```python
from build123d import *

# Parameters (mm, degrees)
BOSS_EXTRUDE3_DEPTH  = 125
SKETCH3_W            = 125
SKETCH3_H            = 92.089876837
BOSS_EXTRUDE5_DEPTH  = 12
CUT_EXTRUDE1_DEPTH   = 126
SKETCH7_W            = 105
SKETCH7_H            = 10
BOSS_EXTRUDE6_DEPTH  = 8
SKETCH8_W            = 105
SKETCH8_H            = 10
BOSS_EXTRUDE7_DEPTH  = 8
SKETCH9_W            = 105
SKETCH9_H            = 73.296024421
CUT_EXTRUDE2_DEPTH   = 16.420201433
SKETCH11_W           = 10
SKETCH11_H           = 73.296024421
CUT_EXTRUDE3_DEPTH   = 6
SKETCH12_W           = 10
SKETCH12_H           = 73.296024421
CUT_EXTRUDE4_DEPTH   = 6
SKETCH13_W           = 105
SKETCH13_H           = 32.67757118
CUT_EXTRUDE6_DEPTH   = 3
SKETCH14_R           = 1.9
CUT_EXTRUDE8_DEPTH   = 6
SKETCH15_R           = 1.9
CUT_EXTRUDE9_DEPTH   = 6
BOSS_EXTRUDE9_REACH  = 117
SKETCH25_W           = 10
SKETCH25_H           = 6
BOSS_EXTRUDE13_DEPTH = 10
CUT_EXTRUDE10_DEPTH  = 1
CUT_EXTRUDE11_DEPTH  = 1


with BuildPart() as part:
    # Sketch1 → Boss-Extrude3 (new body)
    with BuildSketch(Plane(origin=(0, 0, 0), x_dir=(0, 0, -1), z_dir=(1, 0, 0))):
        Polygon((0, 0), (92.089876837, 0), (0, 33.517974046), align=None)
    extrude(amount=-BOSS_EXTRUDE3_DEPTH)

    # Sketch3 → Boss-Extrude5 (add)
    with BuildSketch(Plane.XZ):
        with Locations((-62.5, -46.044938419)):
            Rectangle(SKETCH3_W, SKETCH3_H)
    extrude(amount=BOSS_EXTRUDE5_DEPTH)

    # Sketch6 → Cut-Extrude1 (cut, through all)
    with BuildSketch(Plane.ZY.offset(125)):
        Polygon((-9.396926208, 30.097772613), (-82.692950629, 3.420201433), (-9.396926208, 3.420201433), align=None)
    extrude(amount=-CUT_EXTRUDE1_DEPTH, mode=Mode.SUBTRACT)

    # Sketch7 → Boss-Extrude6 (add)
    with BuildSketch(Plane(origin=(0, 29.597115904, -10.772469209), x_dir=(1, 0, 0), z_dir=(0, 0.939692621, -0.342020143))):
        with Locations((-62.5, 81.536177713)):
            Rectangle(SKETCH7_W, SKETCH7_H)
    extrude(amount=BOSS_EXTRUDE6_DEPTH)

    # Sketch8 → Boss-Extrude7 (add)
    with BuildSketch(Plane(origin=(0, 29.597115904, -10.772469209), x_dir=(1, 0, 0), z_dir=(0, 0.939692621, -0.342020143))):
        with Locations((-62.5, -6.463822287)):
            Rectangle(SKETCH8_W, SKETCH8_H)
    extrude(amount=BOSS_EXTRUDE7_DEPTH)

    # Sketch9 → Cut-Extrude2 (cut, through all)
    with BuildSketch(Plane(origin=(0, 3.420201433, 0), x_dir=(1, 0, 0), z_dir=(0, 1, 0))):
        with Locations((-62.5, 46.044938419)):
            Rectangle(SKETCH9_W, SKETCH9_H)
    extrude(amount=-CUT_EXTRUDE2_DEPTH, mode=Mode.SUBTRACT)

    # Sketch11 → Cut-Extrude3 (cut)
    with BuildSketch(Plane(origin=(0, 3.420201433, 0), x_dir=(1, 0, 0), z_dir=(0, 1, 0))):
        with Locations((-5, 46.044938419)):
            Rectangle(SKETCH11_W, SKETCH11_H)
    extrude(amount=-CUT_EXTRUDE3_DEPTH, mode=Mode.SUBTRACT)

    # Sketch12 → Cut-Extrude4 (cut)
    with BuildSketch(Plane(origin=(0, 3.420201433, 0), x_dir=(1, 0, 0), z_dir=(0, 1, 0))):
        with Locations((-120, 46.044938419)):
            Rectangle(SKETCH12_W, SKETCH12_H)
    extrude(amount=-CUT_EXTRUDE4_DEPTH, mode=Mode.SUBTRACT)

    # Sketch13 → Cut-Extrude6 (cut)
    with BuildSketch(Plane(origin=(0, 0, -9.396926208), x_dir=(-1, 0, 0), z_dir=(0, 0, -1))):
        with Locations((62.5, 13.758987023)):
            Rectangle(SKETCH13_W, SKETCH13_H)
    extrude(amount=-CUT_EXTRUDE6_DEPTH, mode=Mode.SUBTRACT)

    # Sketch14 → Cut-Extrude8 (cut)
    with BuildSketch(Plane(origin=(0, 29.597115904, -10.772469209), x_dir=(1, 0, 0), z_dir=(0, 0.939692621, -0.342020143))):
        with Locations((-6.25, 80.286177713)):
            Circle(SKETCH14_R)
    cut_extrude8 = extrude(amount=-CUT_EXTRUDE8_DEPTH, mode=Mode.SUBTRACT)

    # Mirror1: Cut-Extrude8 across plane
    add(cut_extrude8.mirror(Plane(origin=(-62.5, 0, 0), x_dir=(0, 0, 1), z_dir=(1, 0, 0))), mode=Mode.SUBTRACT)

    # Sketch15 → Cut-Extrude9 (cut)
    with BuildSketch(Plane(origin=(0, 29.597115904, -10.772469209), x_dir=(1, 0, 0), z_dir=(0, 0.939692621, -0.342020143))):
        with Locations((-6.25, -5.213822287)):
            Circle(SKETCH15_R)
    cut_extrude9 = extrude(amount=-CUT_EXTRUDE9_DEPTH, mode=Mode.SUBTRACT)

    # Mirror2: Cut-Extrude9 across plane
    add(cut_extrude9.mirror(Plane(origin=(-62.5, 0, 0), x_dir=(0, 0, 1), z_dir=(1, 0, 0))), mode=Mode.SUBTRACT)

    # Sketch22 → Boss-Extrude9 (add, up to next)
    with BuildSketch(Plane.ZY.offset(10), mode=Mode.PRIVATE) as boss_extrude9_sk1:
        Polygon((-9.396926208, 30.097772613), (-6.396926208, 21.855340354), (-6.396926208, 30.097772613), align=None)
    boss_extrude9_tool1 = extrude(boss_extrude9_sk1.sketch, amount=BOSS_EXTRUDE9_REACH, mode=Mode.PRIVATE) - part.part
    add(boss_extrude9_tool1.solids().sort_by_distance((-10, 27.350295, -7.396926))[0])

    # Sketch25 → Boss-Extrude13 (add)
    with BuildSketch(Plane.XY.offset(-82.692950629)):
        with Locations((-5, 0.420201433)):
            Rectangle(SKETCH25_W, SKETCH25_H)
        with Locations((-120, 0.420201433)):
            Rectangle(SKETCH25_W, SKETCH25_H)
    extrude(amount=BOSS_EXTRUDE13_DEPTH)

    # Sketch26 → Cut-Extrude10 (cut)
    with BuildSketch(Plane(origin=(-10, 0, 0), x_dir=(0, 0, -1), z_dir=(1, 0, 0))):
        Polygon((0, 33.517974046), (9.396926208, 30.097772613), (12.133087354, 37.615313579), (2.736161147, 41.035515012), align=None)
    cut_extrude10 = extrude(amount=-CUT_EXTRUDE10_DEPTH, mode=Mode.SUBTRACT)

    # Sketch27 → Cut-Extrude11 (cut)
    with BuildSketch(Plane(origin=(-10, 0, 0), x_dir=(0, 0, -1), z_dir=(1, 0, 0))):
        Polygon((82.692950629, 3.420201433), (92.089876837, 0), (94.826037984, 7.517540966), (85.429111776, 10.9377424), align=None)
    cut_extrude11 = extrude(amount=-CUT_EXTRUDE11_DEPTH, mode=Mode.SUBTRACT)

    # Mirror3: Cut-Extrude10, Cut-Extrude11 across plane
    add(cut_extrude10.mirror(Plane(origin=(-62.5, 0, 0), x_dir=(0, 0, 1), z_dir=(1, 0, 0))), mode=Mode.SUBTRACT)
    add(cut_extrude11.mirror(Plane(origin=(-62.5, 0, 0), x_dir=(0, 0, 1), z_dir=(1, 0, 0))), mode=Mode.SUBTRACT)


solid = part.part
```
Work out the finished part from the listing and answer in its coordinate system (mm). A direction names the side the tool comes from. Round coordinates to 2 decimals unless told otherwise and drop trailing zeros. Write each loop counter-clockwise with the first axis right and the second up, starting at its lowest first coordinate (ties: lowest second). Pieces come first, ordered by that corner, then holes. Notation, with made-up numbers: (89, 83) - (139, 83) arc R26 cw to (139, 118) - close; hole circle Ø5 at (29.25, 6). An arc over 180 degrees is marked (long way). Return JSON: item names as keys, results as strings. Group by question number.
Q1. Each of these flat-tipped pins is pushed along its axis until it touches: pin 1 Ø11 at (x, y) = (-6.5, 15.5) entering from -Z; pin 2 Ø10.5 at (x, y) = (-61.5, -5.5) entering from -Z; pin 3 Ø5 at (x, z) = (-121, -78) entering from +Y. Where does it stop, or does it pass through?
Q2. The part is cut by section C-C on y = 5. Write down the section's boundary in (x, z), then the cut area to 3 significant figures.
Q3. Find the intervals of material crossed by L1, parallel to X at y = -6, z = -32.5; L2, parallel to Z at x = -27, y = 21; L3, parallel to Z at x = -36.5, y = -5, in increasing order.
Q4. The part is cut by section B-B on x = -87.5. Write down the section's boundary in (y, z).
Q5. The mould has two halves that part along Z. Classify faces 5 (the flat face through (-63, 11, 0)), 6 (the flat face through (-10, 10, -8)), 7 (the cylindrical face through (-6.497, -1.286, -86.975)), 8 (the flat face through (-5, 3.42, -78)): released by +Z, released by -Z, zero draft, split by the parting line, or undercut.
Q6. The part is cut by section A-A on z = -50. Write down the section's boundary in (x, y).
Q7. For faces 1 (the flat face through (-63, -7, -9.397)), 2 (the flat face through (-5, 0, -72.693)), 3 (the flat face through (-114, 6, -89)), 4 (the flat face through (-118.72, -3.51, -84.19)), determine the directions among +Z, -Z, +X, -X, +Y, -Y from which every point of the face is accessible in a straight line to the end or side of a thin tool.
Solved:
{
 "1": {"pin 1": "z = -9.4", "pin 2": "z = -92.09", "pin 3": "y = 3.42"},
 "2": {"outline": "(-125, -9.4) - (-115, -9.4) - (-115, -6.4) - (-10, -6.4) - (-10, -9.4) - (0, -9.4) - (0, 0) - (-125, 0) - close; (-114, -93.91) - (-11, -93.91) - (-11, -83.27) - (-114, -83.27) - close", "area": "1,960 mm²"},
 "3": {"L1": "-125 to -115, -10 to 0", "L2": "-6.4 to 0", "L3": "-92.09 to -82.69, -9.4 to 0"},
 "4": {"outline": "(-12, -92.09) - (0, -92.09) - (7.52, -94.83) - (10.94, -85.43) - (3.42, -82.69) - (-12, -82.69) - close; (-12, -9.4) - (-2.58, -9.4) - (-2.58, -6.4) - (21.86, -6.4) - (37.62, -12.13) - (41.04, -2.74) - (33.52, 0) - (-12, 0) - close"},
 "5": {"face 5": "released by +Z", "face 6": "undercut", "face 7": "undercut", "face 8": "zero draft"},
 "6": {"outline": "(-125, -12) - (-115, -12) - (-115, -2.58) - (-125, -2.58) - close; (-10, -12) - (0, -12) - (0, -2.58) - (-10, -2.58) - close"},
 "7": {"face 1": "-Y", "face 2": "+X, -X, +Y", "face 3": "-Z, -X, +Y", "face 4": "none"}
}
